from build123d import *

# Parameters (mm, degrees)
F1_DEPTH     = 25
F2_R         = 1
F3_T1_DEPTH  = 25
F3_T3_DEPTH  = 25
F3_T5_DEPTH  = 27.1650635095
F3_T7_DEPTH  = 27.5
F3_T9_DEPTH  = 27.5
F3_T11_DEPTH = 27.5
F3_T13_DEPTH = 27.5
F3_T15_DEPTH = 27.1650635095


# Not quite as in the source:
# - a fillet or chamfer that OpenCascade refuses, or shapes differently, is made with other operations: its cross-section is extruded or revolved along the edge and cut away or added


with BuildPart() as f1:
    # F0 (on Top) → F1 (new body)
    with BuildSketch(Plane.XY):
        Polygon((0, 8), (0, 0), (32, 0), (32, 3), (30.2, 3), (3, 3), (3, 5), (32, 5), (32, 8), (19, 8), (19, 9.5), (19.25, 9.5), (19.25, 11.5), (17.5, 11.5), (17.5, 8), (14.5, 8), (14.5, 11.5), (12.75, 11.5), (12.75, 9.5), (13, 9.5), (13, 8), align=None)
        Polygon((30.2, 3), (32, 3), (28.4834179878, 4.5), align=None)
    extrude(amount=F1_DEPTH)

    # F2
    f2_edges = [f1.edges().sort_by_distance(p)[0] for p in [
        (32, 8, 12.5),
        (32, 5, 12.5),
        (32, 0, 12.5),
        (0, 0, 12.5),
        (0, 8, 12.5),
    ]]
    fillet(f2_edges, radius=F2_R)

    # F3: fillet of radius 0.5 on 8 edges, made by hand

    # F3_s2 → F3_t1 (join)
    with BuildSketch(Plane.XY):
        with BuildLine():
            ThreePointArc((14.5, 8.5), (14.6464466094, 8.1464466094), (15, 8))
            Line((15, 8), (14.5, 8))
            Line((14.5, 8), (14.5, 8.5))
        make_face()
    extrude(amount=F3_T1_DEPTH)

    # F3_s4 → F3_t3 (join)
    with BuildSketch(Plane.XY):
        with BuildLine():
            ThreePointArc((17, 8), (17.3535533906, 8.1464466094), (17.5, 8.5))
            Line((17.5, 8.5), (17.5, 8))
            Line((17.5, 8), (17, 8))
        make_face()
    extrude(amount=F3_T3_DEPTH)

    # F3_s6 → F3_t5 (cut)
    with BuildSketch(Plane.XY.offset(-1.0825317547)):
        with BuildLine():
            ThreePointArc((12.75, 9.9330127019), (12.8169872981, 9.6830127019), (13, 9.5))
            Line((13, 9.5), (12.75, 9.5))
            Line((12.75, 9.5), (12.75, 9.9330127019))
        make_face()
    extrude(amount=F3_T5_DEPTH, mode=Mode.SUBTRACT)

    # F3_s8 → F3_t7 (cut)
    with BuildSketch(Plane.XY.offset(-1.25)):
        with BuildLine():
            ThreePointArc((12.75, 11), (12.8964466094, 11.3535533906), (13.25, 11.5))
            Line((13.25, 11.5), (12.75, 11.5))
            Line((12.75, 11.5), (12.75, 11))
        make_face()
    extrude(amount=F3_T7_DEPTH, mode=Mode.SUBTRACT)

    # F3_s10 → F3_t9 (cut)
    with BuildSketch(Plane.XY.offset(-1.25)):
        with BuildLine():
            ThreePointArc((14, 11.5), (14.3535533906, 11.3535533906), (14.5, 11))
            Line((14.5, 11), (14.5, 11.5))
            Line((14.5, 11.5), (14, 11.5))
        make_face()
    extrude(amount=F3_T9_DEPTH, mode=Mode.SUBTRACT)

    # F3_s12 → F3_t11 (cut)
    with BuildSketch(Plane.XY.offset(-1.25)):
        with BuildLine():
            ThreePointArc((17.5, 11), (17.6464466094, 11.3535533906), (18, 11.5))
            Line((18, 11.5), (17.5, 11.5))
            Line((17.5, 11.5), (17.5, 11))
        make_face()
    extrude(amount=F3_T11_DEPTH, mode=Mode.SUBTRACT)

    # F3_s14 → F3_t13 (cut)
    with BuildSketch(Plane.XY.offset(-1.25)):
        with BuildLine():
            ThreePointArc((18.75, 11.5), (19.1035533906, 11.3535533906), (19.25, 11))
            Line((19.25, 11), (19.25, 11.5))
            Line((19.25, 11.5), (18.75, 11.5))
        make_face()
    extrude(amount=F3_T13_DEPTH, mode=Mode.SUBTRACT)

    # F3_s16 → F3_t15 (cut)
    with BuildSketch(Plane.XY.offset(-1.0825317547)):
        with BuildLine():
            ThreePointArc((19.25, 9.9330127019), (19.1830127019, 9.6830127019), (19, 9.5))
            Line((19, 9.5), (19.25, 9.5))
            Line((19.25, 9.5), (19.25, 9.9330127019))
        make_face()
    extrude(amount=F3_T15_DEPTH, mode=Mode.SUBTRACT)


solid = f1.part
Part model, mm, in its own coordinate system. A direction names the side the tool comes from. Coordinates: 2 decimals unless noted, no trailing zeros. Loops run counter-clockwise (first coordinate to the right, second up) from the corner with the lowest first, then second, coordinate; pieces in that order, holes last. Notation, with made-up numbers: M -26.75,65.5 L 30.25,65.5 A25 ccw 30.25,101.5 Z; hole C -33,50.5 d10. An arc over 180 degrees is marked long. Use a Markdown table: item, result. Add a question column.
Q1. Mould opens along X. For faces 1 (the flat face through (17, 3, 12)), 2 (the cylindrical face through (0.285, 0.301, 12.675)), 3 (the flat face through (7, 8, 12)) say: +X half, -X half, draft (parallel to the pull), parting line (faces both ways), or undercut.
Q2. Probe L1, parallel to Y at x = 8.5, z = 15; L2, parallel to X at y = 9, z = 5.5; L3, parallel to Y at x = 13.5, z = 20.5. List the from-to ranges inside material, lowest first.
Q3. Cut at B-B (x = 21). Write the cut outline in (y, z).
Q4. Pin check, flat tips, straight feed: P1, Ø1.2, axis at y = 10, z = 13, coming from the +X side; P2, Ø0.6, axis at x = 15.5, z = 8, coming from the +Y side; P3, Ø3, axis at y = 9, z = 7.5, coming from the -X side. Stop position of each tip, or through.
Q5. Which spindle directions (+Z, -Z, +X, -X, +Y, -Y) get a long thin tool onto all of the face, cutting with end or side? Do faces 4 (the cylindrical face through (31.699, 5.285, 12.675)), 5 (the flat face through (3, 4, 12)), 6 (the flat face through (14.5, 10, 12)), 7 (the flat face through (19.25, 10.5, 12.3)). Say none if no direction does.
Q6. Cut at A-A (y = 10.5). Write the cut outline in (x, z).
Worked out:
| question | item | result |
|---|---|---|
| 1 | face 1 | undercut |
| 1 | face 2 | -X half |
| 1 | face 3 | draft |
| 2 | L1 | y = 0 to 3, 5 to 8 |
| 2 | L2 | x = 13 to 14.5, 17.5 to 19 |
| 2 | L3 | y = 0 to 3, 5 to 11.5 |
| 3 | outline | M 0,0 L 3,0 L 3,25 L 0,25 Z; M 5,0 L 8,0 L 8,25 L 5,25 Z |
| 4 | P1 | stops at x = 19.25 |
| 4 | P2 | stops at y = 8 |
| 4 | P3 | stops at x = 0.13 |
| 5 | face 4 | +Z, -Z, +X |
| 5 | face 5 | +Z, -Z |
| 5 | face 6 | +Z, -Z, +Y |
| 5 | face 7 | +Z, -Z, +X, +Y |
| 6 | outline | M 12.75,0 L 14.5,0 L 14.5,25 L 12.75,25 Z; M 17.5,0 L 19.25,0 L 19.25,25 L 17.5,25 Z |
